Input: dimensioned drawing with shaded views. Units: mm. Origin: part minimum x, y, z. Round coordinates to 2 decimals unless told otherwise and drop trailing zeros. Order: outer loops, then holes, each group sorted by start corner. A loop starts at its lowest first (then second) coordinate and runs counter-clockwise, first axis right, second up. Notation, with made-up numbers: M 51,-36.75 L 80,-36.75 A32 ccw 80,-9.75 Z; hole C 7.25,18 d3. An arc over 180 degrees is marked long. One line per question, with ' | ' between items.
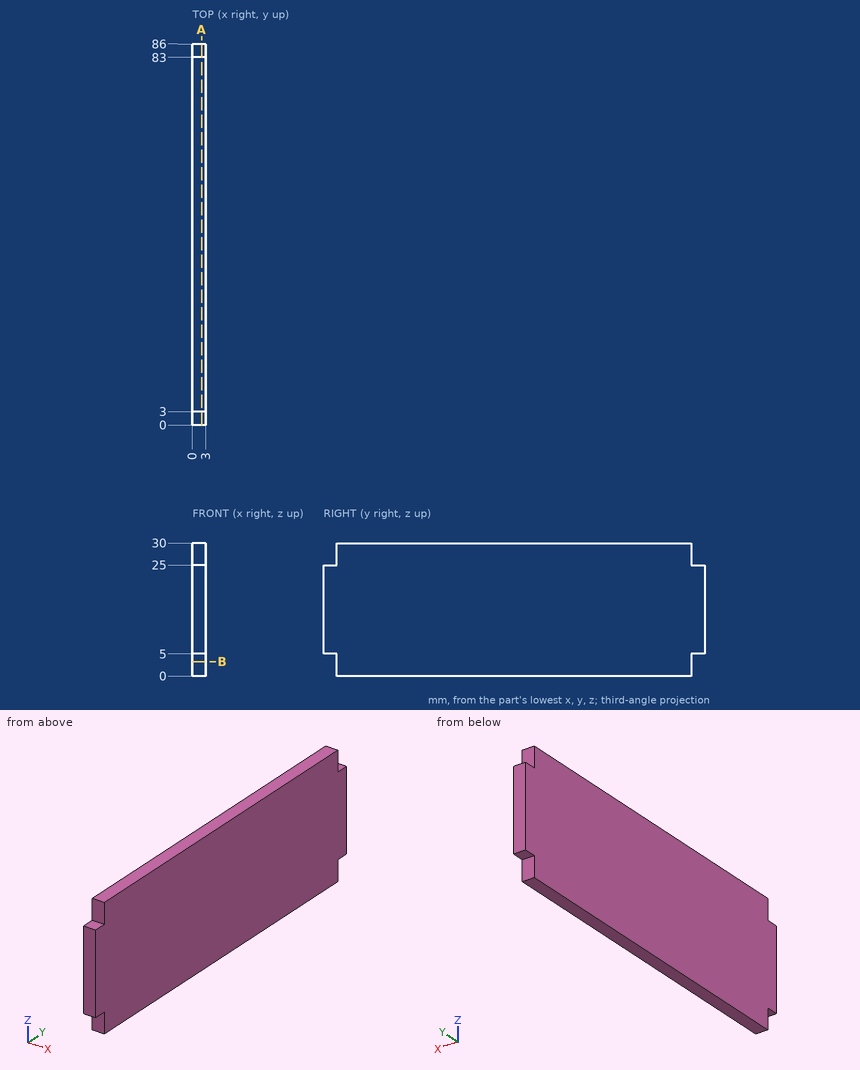
Item 1: Section query A-A, the plane x = 2.1. Return loops of the section in (y, z).
Report:
outline: M 0,5 L 3,5 L 3,0 L 83,0 L 83,5 L 86,5 L 86,25 L 83,25 L 83,30 L 3,30 L 3,25 L 0,25 Z
Item 2: First-contact query: pin 1 (0.9 mm diameter, centred on x = 1, z = 3, fed in from +Y); pin 2 (0.9 mm diameter, centred on x = 1.5, y = 1.5, fed in from +Z); pin 3 (1.5 mm diameter, centred on x = 1, y = 84.5, fed in from -Z). Flat tips, straight axial feed; report the tip coordinate or a pass-through.
Report:
pin 1: y = 83 | pin 2: z = 25 | pin 3: z = 5
Item 3: Section query B-B, the plane z = 3.25. Return loops of the section in (x, y), plus the area to 3 significant figures.
Report:
outline: M 0,3 L 3,3 L 3,83 L 0,83 Z | area: 240 mm²
Item 4: Line query: line 1 along Y through (x, z) = (2.35, 2.25). Output: solid intervals per line, ascending. Write a range as from..to.
Report:
line 1: 3..83
